Autodesk Inventor part; units mm, degrees
ref_plane "YZ Plane" through (0, 0, 0) normal (1, 0, 0) x (0, 1, 0)
ref_plane "XZ Plane" through (0, 0, 0) normal (0, 1, 0) x (-1, 0, 0)
ref_plane "XY Plane" through (0, 0, 0) normal (0, 0, 1) x (1, 0, 0)
sketch "Sketch1" plane through (0, 0, 0) normal (0, 0, 1) x (1, 0, 0)
  line L0 (0, 0) -> (1200, 0)
  line L1 (1200, 0) -> (1200, 450)
  line L2 (1200, 450) -> (0, 450)
  line L3 (0, 450) -> (0, 0)
  line L4 (3, 447) -> (1197, 447)
  line L5 (1197, 447) -> (1197, 3)
  line L6 (1197, 3) -> (3, 3)
  line L7 (3, 3) -> (3, 447)
  dimension "d8" = 1200
  dimension "d9" = 450
  dimension "d10" = 3
extrude "Extrusion2" add sketch "Sketch1" against normal blind 40
extrude "Extrusion3" add sketch "Sketch1" against normal blind 3 contours L3 L2 L1 L0 | L4 L5 L6 L7
sketch "Sketch2" plane through (0, 450, -40) normal (0, 1, 0) x (1, 0, 0)
  line L0 (0, -40) -> (0, 0)
  line L1 (1200, -40) -> (0, -40)
  line L2 (1200, -40) -> (1200, 0)
  point P0 (15, -25)
  point P1 (1185, -25)
  dimension "d22" = 15
  dimension "d23" = 15
  dimension "d24" = 15
  dimension "d25" = 15
hole "Hole1" at (15, 450, -15) at (1185, 450, -15) direction (0, -1, 0) diameter 3.81 end through all
sketch "Sketch3" plane through (0, 0, -40) normal (-1, 0, 0) x (0, 0, 1)
  line L0 (40, 450) -> (40, 0)
  line L1 (40, 0) -> (0, 0)
  line L2 (40, 450) -> (0, 450)
  point P0 (25, 15)
  point P1 (25, 435)
  dimension "d26" = 15
  dimension "d27" = 15
  dimension "d28" = 15
  dimension "d29" = 15
hole "Hole2" at (0, 15, -15) at (0, 435, -15) direction (1, 0, 0) diameter 3.81 end through all
equation "\"d8\" = Width"
equation "\"d9\" = Depth"
equation "\"d10\" = Thickness"
equation "\"d11\" = Height"
equation "\"d13\" = Thickness"
equation "\"Width\" = 1200"
equation "\"Thickness\" = 3"
equation "\"Depth\" = 450"
equation "\"Height\" = 40"
equation "\"HoleDistance\" = 15"
properties part number "shelf120"
Geometry: final body of the model. Coordinates: model frame, mm. A direction names the side the tool comes from. Give positions to 0.01 mm unless a question says otherwise; leave off trailing zeros. Order: outer loops, then holes, each group sorted by start corner. A loop starts at its lowest first (then second) coordinate and runs counter-clockwise, first axis right, second up. Notation, with made-up numbers: (58.25, -26.5) -> (102.25, -26.5) arc R10 ccw to (102.25, -13.5) -> close; hole circle Ø7 at (-23, -26). An arc over 180 degrees is marked (long way). Answer as a JSON object with one key per item and string values.
Q1. Section A-A (z = -27). Output: boundary loops of the cut face in (x, y).
Entries:
{"outline": "(0, 0) -> (1200, 0) -> (1200, 450) -> (0, 450) -> close; hole (3, 3) -> (1197, 3) -> (1197, 447) -> (3, 447) -> close"}
Q2. Draft query along Y for faces 3 (the flat face through (608, 3, -21)), 4 (the flat face through (608, 450, -20)), 5 (the flat face through (0, 228, -20)), 6 (the flat face through (592, 0, -20)). Return one class per face: released by +Y, released by -Y, zero draft, split by the parting line, or undercut.
Entries:
{"face 3": "undercut", "face 4": "released by +Y", "face 5": "zero draft", "face 6": "released by -Y"}
Q3. Section B-B (x = 906). Output: boundary loops of the cut face in (y, z), plus the area to 3 significant figures.
Entries:
{"outline": "(0, -40) -> (3, -40) -> (3, -3) -> (447, -3) -> (447, -40) -> (450, -40) -> (450, 0) -> (0, 0) -> close", "area": "1,570 mm^2"}
Q4. Section C-C (y = 156). Output: boundary loops of the cut face in (x, z).
Entries:
{"outline": "(0, -40) -> (3, -40) -> (3, -3) -> (1197, -3) -> (1197, -40) -> (1200, -40) -> (1200, 0) -> (0, 0) -> close"}
Q5. Access query for faces 1 (the flat face through (592, 447, -21)), 2 (the flat face through (592, 228, 0)). Directions: +Z, -Z, +X, -X, +Y, -Y. A direction counts if a zero-diameter tool reaches every point of the face in a straight line with its end or side. Return the directions, or none.
Entries:
{"face 1": "-Z", "face 2": "+Z, +X, -X, +Y, -Y"}
Q6. Material intervals for probe 1 along Y at (x, z) = (2.1, -15) (3 decimals); probe 2 along X at (y, z) = (0.8, -15) (3 decimals); probe 3 along X at (y, z) = (32, -20), sorted ascending.
Entries:
{"probe 1": "y = 0 to 13.095, 16.905 to 433.095, 436.905 to 450", "probe 2": "x = 0 to 13.095, 16.905 to 1183.095, 1186.905 to 1200", "probe 3": "x = 0 to 3, 1197 to 1200"}
Q7. First-contact query: pin 1 (4 mm diameter, centred on x = 472.5, y = 306, fed in from -Z). Flat tip, straight axial feed; report the tip coordinate or a pass-through.
Entries:
{"pin 1": "stops at z = -3"}
